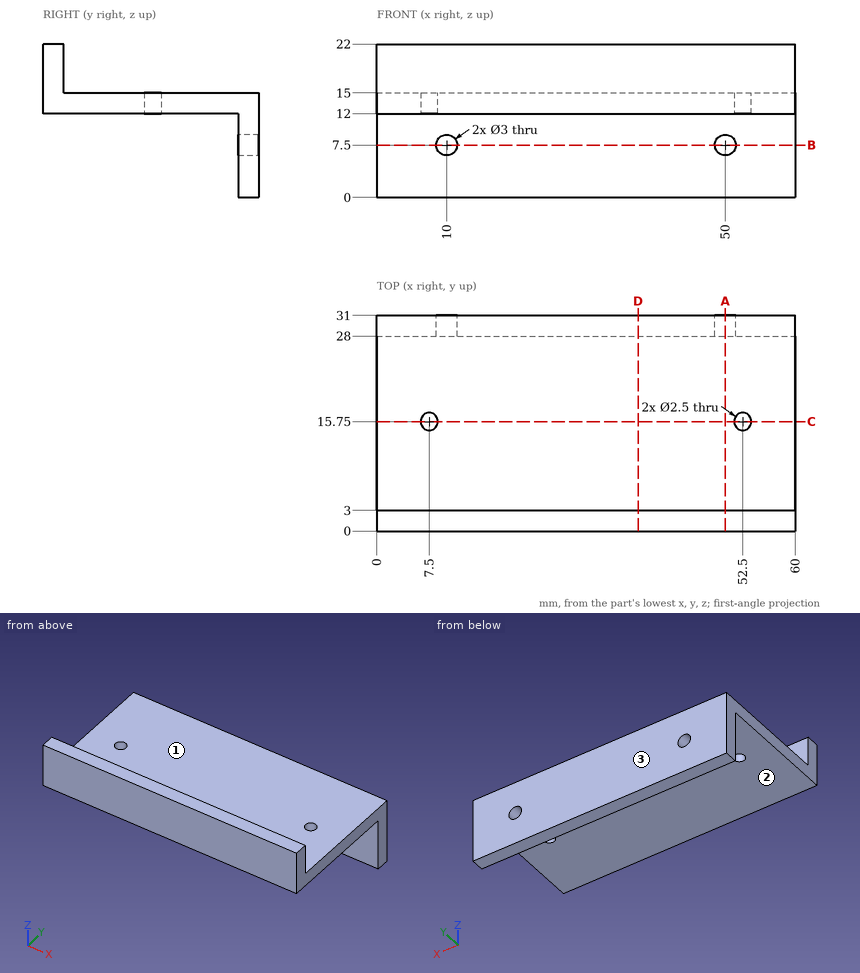
Geometry: see drawing. Coordinates: mm, zero at the bounding-box minimum. A direction names the side the tool comes from. Give positions to 0.01 mm unless a question says otherwise; leave off trailing zeros. Write each loop counter-clockwise with the first axis right and the second up, starting at its lowest first coordinate (ties: lowest second). Pieces come first, ordered by that corner, then holes. Notation, with made-up numbers: M 59,29.5 L 80,29.5 A25 ccw 80,42.5 Z; hole C 46.25,61.5 d9. An arc over 180 degrees is marked long. Return JSON: item names as keys, results as strings. Group by question number.
1) First-contact query: pin 1 Ø3.5 at (x, z) = (30.5, 19.5) entering from +Y; pin 2 Ø2 at (x, y) = (52.5, 15.75) entering from +Z; pin 3 Ø10 at (x, y) = (19.5, 18) entering from -Z; pin 4 Ø13 at (x, z) = (30, 5) entering from -Y. Flat tips, straight axial feed; report the tip coordinate or a pass-through.
2) Cut plane C-C, the plane y = 15.75. Output: boundary loops of the cut face in (x, z).
3) Cut plane D-D, the plane x = 37.5. Output: boundary loops of the cut face in (y, z).
4) Cut plane B-B, the plane z = 7.5. Output: boundary loops of the cut face in (x, y).
5) Cut plane A-A, the plane x = 50. Output: boundary loops of the cut face in (y, z), then the cut area to 3 significant figures.
6) Ray query, L1, parallel to X at y = 28.85, z = 7.5; L2, parallel to Y at x = 7.5, z = 13.65; L3, parallel to Z at x = 12, y = 21. Return the intervals inside material, ascending.
7) Set-up query: the marked faces 1, 2 and 3. Return all of +Z, -Z, +X, -X, +Y, -Y with unobstructed straight access to the full face (end or side cutting, diameter ignored); none if empty.
Data:
{
 "1": {"pin 1": "stops at y = 3", "pin 2": "passes through", "pin 3": "stops at z = 12", "pin 4": "stops at y = 28"},
 "2": {"outline": "M 0,12 L 6.25,12 L 6.25,15 L 0,15 Z; M 8.75,12 L 51.25,12 L 51.25,15 L 8.75,15 Z; M 53.75,12 L 60,12 L 60,15 L 53.75,15 Z"},
 "3": {"outline": "M 0,12 L 28,12 L 28,0 L 31,0 L 31,15 L 3,15 L 3,22 L 0,22 Z"},
 "4": {"outline": "M 0,28 L 8.5,28 L 8.5,31 L 0,31 Z; M 11.5,28 L 48.5,28 L 48.5,31 L 11.5,31 Z; M 51.5,28 L 60,28 L 60,31 L 51.5,31 Z"},
 "5": {"outline": "M 0,12 L 28,12 L 28,9 L 31,9 L 31,15 L 3,15 L 3,22 L 0,22 Z; M 28,0 L 31,0 L 31,6 L 28,6 Z", "area": "141 mm²"},
 "6": {"L1": "x = 0 to 8.5, 11.5 to 48.5, 51.5 to 60", "L2": "y = 0 to 14.5, 17 to 31", "L3": "z = 12 to 15"},
 "7": {"face 1": "+Z, +X, -X, +Y", "face 2": "-Z, +X, -X, -Y", "face 3": "+Z, -Z, +X, -X, +Y"}
}
